Autodesk Fusion 360 part; units mm, degrees
sketch "Sketch1" plane through (0, 0, 0) normal (0, 0, 1) x (1, 0, 0)
  line L0 (0, 0) -> (37.5, 0)
  line L1 (37.5, 0) -> (37.5, 32)
  line L2 (37.5, 32) -> (0, 32)
  line L3 (0, 32) -> (0, 0)
  dimension "d1" = 37.5
  dimension "d2" = 32
extrude "Extrude1" add sketch "Sketch1" along normal blind 2.5
sketch "Sketch2" plane through (0, 0, 2.5) normal (0, 0, 1) x (-1, 0, 0)
  line L0 (0, -32) -> (0, 0)
  line L1 (0, 0) -> (-37.5, 0)
  line L2 (-37.5, 0) -> (-37.5, -32)
  line L3 (-37.5, -32) -> (0, -32)
  circle A0 centre (-18.75, -29.75) radius 1.25
  dimension "d5" = 2.5
  dimension "d6" = 18.75
  dimension "d7" = 2.25
extrude "Extrude2" cut sketch "Sketch2" against normal blind 3 contours A0
sketch "Sketch3" plane through (0, 0, 2.5) normal (0, 0, 1) x (-1, 0, 0)
  circle A0 centre (-18.75, -29.75) radius 1.25
  line L0 (0, -32) -> (0, 0)
  line L1 (0, 0) -> (-37.5, 0)
  line L2 (-37.5, 0) -> (-37.5, -32)
  line L3 (-37.5, -32) -> (0, -32)
  circle A1 centre (-18.75, -2.25) radius 1.25
  dimension "d10" = 2.5
  dimension "d11" = 27.5
  dimension "d12" = 18.75
extrude "Extrude3" cut sketch "Sketch3" against normal blind 3 contours A1
sketch "Sketch4" plane through (0, 0, 2.5) normal (0, 0, 1) x (-1, 0, 0)
  circle A0 centre (-18.75, -2.25) radius 1.25
  circle A1 centre (-18.75, -29.75) radius 1.25
  line L0 (0, -32) -> (0, 0)
  line L1 (0, 0) -> (-37.5, 0)
  line L2 (-37.5, 0) -> (-37.5, -32)
  line L3 (-37.5, -32) -> (0, -32)
  line L4 (-12.75, -27.5) -> (-24.75, -27.5)
  line L5 (-24.75, -27.5) -> (-24.75, -4.5)
  line L6 (-24.75, -4.5) -> (-12.75, -4.5)
  line L7 (-12.75, -4.5) -> (-12.75, -27.5)
  dimension "d15" = 23
  dimension "d16" = 12
  dimension "d17" = 6
  dimension "d18" = 2.25
extrude "Extrude4" cut sketch "Sketch4" against normal blind 3 contours L4 L5 L6 L7
sketch "Sketch5" plane through (37.5, 0, 0) normal (1, 0, 0) x (0, 1, 0)
  line L0 (0, 0) -> (32, 0)
  line L1 (32, 0) -> (32, 2.5)
  line L2 (32, 2.5) -> (0, 2.5)
  line L3 (0, 2.5) -> (0, 0)
  line L4 (25.5, 2.5) -> (14, 2.5)
  line L5 (14, 2.5) -> (14, 0)
  line L6 (14, 0) -> (25.5, 0)
  line L7 (25.5, 0) -> (25.5, 2.5)
  point P0 (27.5, 2.5)
  dimension "d21" = 11.5
  dimension "d22" = 2
extrude "Extrude5" cut sketch "Sketch5" against normal blind 3 contours L0 L2 L3 L5 | L0 L1 L2 L7
sketch "Sketch6" plane through (0, 0, 0) normal (-1, 0, 0) x (0, -1, 0)
  line L0 (-32, 0) -> (0, 0)
  line L1 (0, 0) -> (0, 2.5)
  line L2 (0, 2.5) -> (-32, 2.5)
  line L3 (-32, 2.5) -> (-32, 0)
  line L4 (-25.5, 2.5) -> (-14, 2.5)
  line L5 (-14, 2.5) -> (-14, 0)
  line L6 (-14, 0) -> (-25.5, 0)
  line L7 (-25.5, 0) -> (-25.5, 2.5)
  point P0 (-27.5, 2.5)
  dimension "d25" = 11.5
  dimension "d26" = 2
extrude "Extrude6" cut sketch "Sketch6" against normal blind 3 contours L0 L2 L3 L7 | L0 L1 L2 L5
sketch "Sketch7" plane through (0, 0, 2.5) normal (0, 0, 1) x (-1, 0, 0)
  line L0 (-3, -25.5) -> (0, -25.5)
  line L1 (0, -25.5) -> (0, -14)
  line L2 (0, -14) -> (-3, -14)
  line L3 (-3, -14) -> (-3, 0)
  line L4 (-3, 0) -> (-34.5, 0)
  line L5 (-34.5, 0) -> (-34.5, -14)
  line L6 (-34.5, -14) -> (-37.5, -14)
  line L7 (-37.5, -14) -> (-37.5, -25.5)
  line L8 (-37.5, -25.5) -> (-34.5, -25.5)
  line L9 (-34.5, -25.5) -> (-34.5, -32)
  line L10 (-34.5, -32) -> (-3, -32)
  line L11 (-3, -32) -> (-3, -25.5)
  circle A0 centre (-18.75, -29.75) radius 1.25
  circle A1 centre (-18.75, -2.25) radius 1.25
  line L12 (-24.75, -27.5) -> (-24.75, -4.5)
  line L13 (-24.75, -4.5) -> (-12.75, -4.5)
  line L14 (-12.75, -4.5) -> (-12.75, -27.5)
  line L15 (-12.75, -27.5) -> (-24.75, -27.5)
  spline S0 degree 5 poles (-3, -28.75) (-3.63, -28.9965) (-4.89, -29.468) (-6.78, -30.1106) (-9.3, -30.8362) (-12.45, -31.5094) (-15.6, -31.9281) (-18.75, -32.0715) (-21.9, -31.9281) (-25.05, -31.5094) (-28.2, -30.8362) (-30.72, -30.1106) (-32.61, -29.468) (-33.87, -28.9965) (-34.5, -28.75) knots 0 0 0 0 0 0 0.1 0.2 0.3 0.4 0.5 0.6 0.7 0.8 0.9 1 1 1 1 1 1
  point P0 (-18.75, -32)
extrude "Extrude7" cut sketch "Sketch7" against normal blind 3 contours L10 L11 S0 | L9 L10 S0
fillet "Fillet1" radius 1 1 edges at (34.5, 28.75, 1.25)
fillet "Fillet2" radius 1 1 edges at (3, 28.75, 1.25)
sketch "Sketch8" plane through (0, 0, 2.5) normal (0, 0, 1) x (-1, 0, 0)
  spline S0 degree 3 poles (-3, -28.063) (-3, -28.1932) (-3.0254, -28.3222) (-3.1243, -28.5631) (-3.1968, -28.6728) (-3.3388, -28.8166) (-3.3947, -28.8622) (-3.5154, -28.9407) (-3.5797, -28.9732) (-3.647, -28.9986) knots 0 0 0 0 0.039064 0.039064 0.078129 0.078129 0.099711 0.099711 0.121294 0.121294 0.121294 0.121294
  line L0 (-3, -28.063) -> (-3, -25.5)
  line L1 (-3, -25.5) -> (0, -25.5)
  line L2 (0, -25.5) -> (0, -14)
  line L3 (0, -14) -> (-3, -14)
  line L4 (-3, -14) -> (-3, 0)
  line L5 (-3, 0) -> (-34.5, 0)
  line L6 (-34.5, 0) -> (-34.5, -14)
  line L7 (-34.5, -14) -> (-37.5, -14)
  line L8 (-37.5, -14) -> (-37.5, -25.5)
  line L9 (-37.5, -25.5) -> (-34.5, -25.5)
  line L10 (-34.5, -25.5) -> (-34.5, -28.063)
  spline S1 degree 3 poles (-33.853, -28.9986) (-33.9748, -28.9527) (-34.0865, -28.8834) (-34.277, -28.7058) (-34.354, -28.5993) (-34.4385, -28.4156) (-34.4615, -28.3472) (-34.4922, -28.2067) (-34.5, -28.1349) (-34.5, -28.063) knots 0 0 0 0 0.039064 0.039064 0.078129 0.078129 0.099711 0.099711 0.121294 0.121294 0.121294 0.121294
  spline S2 degree 5 poles (-33.853, -28.9986) (-33.3524, -29.1875) (-32.2218, -29.5986) (-30.4612, -30.1847) (-28.0706, -30.8638) (-25.05, -31.5094) (-22.53, -31.8444) (-20.64, -31.9717) (-19.38, -32) (-18.75, -32) knots -0.979459 -0.979459 -0.979459 -0.979459 -0.979459 -0.979459 -0.9 -0.8 -0.7 -0.6 -0.5 -0.5 -0.5 -0.5 -0.5 -0.5
  spline S3 degree 5 poles (-18.75, -32) (-18.12, -32) (-16.86, -31.9717) (-14.97, -31.8444) (-12.45, -31.5094) (-9.4294, -30.8638) (-7.0388, -30.1847) (-5.2782, -29.5986) (-4.1476, -29.1875) (-3.647, -28.9986) knots -0.5 -0.5 -0.5 -0.5 -0.5 -0.5 -0.4 -0.3 -0.2 -0.1 -0.020541 -0.020541 -0.020541 -0.020541 -0.020541 -0.020541
  circle A0 centre (-18.75, -29.75) radius 1.25
  circle A1 centre (-18.75, -2.25) radius 1.25
  line L11 (-24.75, -27.5) -> (-24.75, -4.5)
  line L12 (-24.75, -4.5) -> (-12.75, -4.5)
  line L13 (-12.75, -4.5) -> (-12.75, -27.5)
  line L14 (-12.75, -27.5) -> (-24.75, -27.5)
  spline S4 degree 5 poles (-3, -10.0882) (-3.192, -9.5306) (-3.5896, -8.4564) (-4.2262, -6.9676) (-5.156, -5.2287) (-6.4542, -3.4672) (-7.8881, -2.1125) (-9.4541, -1.1457) (-11.1442, -0.5279) (-12.9429, -0.19) (-14.8281, -0.0435) (-16.7736, -0.0017) (-18.75, 0.0027) (-20.7264, -0.0017) (-22.6719, -0.0435) (-24.5571, -0.19) (-26.3558, -0.5279) (-28.0459, -1.1457) (-29.6119, -2.1125) (-31.0458, -3.4672) (-32.344, -5.2287) (-33.2738, -6.9676) (-33.9104, -8.4564) (-34.308, -9.5306) (-34.5, -10.0882) knots 0 0 0 0 0 0 0.05 0.1 0.15 0.2 0.25 0.3 0.35 0.4 0.45 0.5 0.55 0.6 0.65 0.7 0.75 0.8 0.85 0.9 0.95 1 1 1 1 1 1
  point P0 (-10, -1)
  point P1 (-18.75, 0)
  point P2 (-27.5, -1)
  dimension "d35" = 8.75
  dimension "d36" = 8.75
  dimension "d37" = 1
  dimension "d38" = 1
extrude "Extrude8" cut sketch "Sketch8" against normal blind 3 contours L4 L5 S4 | L5 L6 S4
fillet "Fillet3" radius 4 1 edges at (3, 10.0882, 1.25)
fillet "Fillet4" radius 4 1 edges at (34.5, 10.0882, 1.25)
Geometry: final body of the model. Coordinates: model frame, mm. A direction names the side the tool comes from. Give positions to 0.01 mm unless a question says otherwise; leave off trailing zeros. Write each loop counter-clockwise with the first axis right and the second up, starting at its lowest first coordinate (ties: lowest second). Pieces come first, ordered by that corner, then holes.
(1) Cut plane B-B, the plane y = 18.5. Return loops of the section in (x, z), then the cut area to 4 significant figures.
(2) Cut plane A-A, the plane y = 13.5. Return loops of the section in (x, z), then the cut area to 4 significant figures.
(3) Ray query, line 1 (Y direction, x = 18.75, z = 0.75); line 2 (X direction, y = 16.5, z = 1.35); line 3 (Y direction, x = 2.5, z = 1.55). Return the intervals inside material, ascending.
(4) Access query for faces 1 (the flat face through (34.5, 12, 1)), 2 (the flat face through (1, 14, 1)), 3 (the flat face through (24.75, 16, 1)), 4 (the flat face through (34.5, 27, 1)). Directions: +Z, -Z, +X, -X, +Y, -Y. A direction counts if a zero-diameter tool reaches every point of the face in a straight line with its end or side. Return the directions, or none.
(5) Mould query, pull axis X, two halves, no side actions, for faces 5 (the flat face through (19, 4.5, 1)), 6 (the flat face through (1, 25.5, 1)), 7 (the flat face through (37.5, 20, 1)), 8 (the cylindrical face through (18.078, 28.696, 1.268)). Classes: released by +X, released by -X, zero draft, split by the parting line, or undercut.
(6) First-contact query: P1, Ø1.3, axis at y = 12, z = 0.5, coming from the -X side; P2, Ø5, axis at x = 20.5, y = 26.5, coming from the -Z side; P3, Ø1.2, axis at x = 1.5, z = 1, coming from the +Y side; P4, Ø0.8, axis at x = 1.5, z = 1, coming from the -Y side. Flat tips, straight axial feed; report the tip coordinate or a pass-through.
(7) Cut plane C-C, the plane z = 1.2. Give the number of separate pieces and of enclosed holes in the cut face, then the cut area to 3 significant figures.
Values follow:
1. outline: (0, 0) - (12.75, 0) - (12.75, 2.5) - (0, 2.5) - close; (24.75, 0) - (37.5, 0) - (37.5, 2.5) - (24.75, 2.5) - close
1. area: 63.75 mm2
2. outline: (3, 0) - (12.75, 0) - (12.75, 2.5) - (3, 2.5) - close; (24.75, 0) - (34.5, 0) - (34.5, 2.5) - (24.75, 2.5) - close
2. area: 48.75 mm2
3. line 1: y = 0 to 1, 3.5 to 4.5, 27.5 to 28.5, 31 to 32
3. line 2: x = 0 to 12.75, 24.75 to 37.5
3. line 3: y = 14 to 25.5
4. face 1: +Z, -Z, +X, -Y
4. face 2: +Z, -Z, -X, -Y
4. face 3: +Z, -Z
4. face 4: +Z, -Z, +X, +Y
5. face 5: undercut
5. face 6: zero draft
5. face 7: released by +X
5. face 8: undercut
6. P1: stops at x = 3
6. P2: stops at z = 0
6. P3: stops at y = 25.5
6. P4: stops at y = 14
7. separate pieces: 1
7. enclosed holes: 3
7. area: 693 mm2
